from build123d import *

# Parameters (mm, degrees)
F0_R     = 3.96875
F1_DEPTH = 12.7
F4_DEPTH = 12.7
F6_DEPTH = 12.7
F8_DEPTH = 330.2


with BuildPart() as f1:
    # F0 (on Top) → F1 (new body)
    with BuildSketch(Plane.XY):
        Polygon((342.9, 76.2), (-342.9, 76.2), (-377.825, 31.75), (-377.825, -31.75), (-342.9, -76.2), (342.9, -76.2), align=None)
        with Locations((-317.5, -63.5)):
            Circle(F0_R, mode=Mode.SUBTRACT)
        with Locations((-190.5, -63.5)):
            Circle(F0_R, mode=Mode.SUBTRACT)
        with Locations((-63.5, -63.5)):
            Circle(F0_R, mode=Mode.SUBTRACT)
        with Locations((63.5, -63.5)):
            Circle(F0_R, mode=Mode.SUBTRACT)
        with Locations((190.5, -63.5)):
            Circle(F0_R, mode=Mode.SUBTRACT)
        with Locations((317.5, -63.5)):
            Circle(F0_R, mode=Mode.SUBTRACT)
        with Locations((-317.5, 63.5)):
            Circle(F0_R, mode=Mode.SUBTRACT)
        with Locations((-190.5, 63.5)):
            Circle(F0_R, mode=Mode.SUBTRACT)
        with Locations((-63.5, 63.5)):
            Circle(F0_R, mode=Mode.SUBTRACT)
        with Locations((63.5, 63.5)):
            Circle(F0_R, mode=Mode.SUBTRACT)
        with Locations((190.5, 63.5)):
            Circle(F0_R, mode=Mode.SUBTRACT)
        with Locations((317.5, 63.5)):
            Circle(F0_R, mode=Mode.SUBTRACT)
    extrude(amount=F1_DEPTH)

    # F3 (on plane+point) → F4 (join)
    with BuildSketch(Plane.YZ.offset(-342.9)):
        Polygon((76.2, 63.5), (-76.2, 63.5), (-76.2, 12.7), (-31.75, 12.7), (-31.75, 50.8), (31.75, 50.8), (31.75, 12.7), (76.2, 12.7), align=None)
    extrude(amount=F4_DEPTH)

    # F5 (on face) → F6 (join)
    with BuildSketch(Plane.YZ.offset(342.9)):
        Polygon((-76.2, 63.5), (-76.2, 12.7), (-31.75, 12.7), (-31.75, 50.8), (31.75, 50.8), (31.75, 12.7), (76.2, 12.7), (76.2, 63.5), align=None)
    extrude(amount=-F6_DEPTH)

    # F7 (on Right) → F8 (join, symmetric)
    with BuildSketch(Plane.YZ):
        Polygon((69.85, 12.7), (76.2, 12.7), (76.2, 57.15), (71.4375, 57.15), (71.4375, 55.5625), (74.6125, 55.5625), (74.6125, 44.45), (69.85, 44.45), align=None)
        Polygon((-71.4375, 57.15), (-76.2, 57.15), (-76.2, 12.7), (-69.85, 12.7), (-69.85, 44.45), (-74.6125, 44.45), (-74.6125, 55.5625), (-71.4375, 55.5625), align=None)
    extrude(amount=F8_DEPTH, both=True)


solid = f1.part
For this review, take the finished solid that the model builds, in its own axes (mm). A direction names the side the tool comes from. Round coordinates to 2 decimals unless told otherwise and drop trailing zeros. Write each loop counter-clockwise with the first axis right and the second up, starting at its lowest first coordinate (ties: lowest second). Pieces come first, ordered by that corner, then holes. Notation, with made-up numbers: (58, -18.75) - (111, -18.75) arc R10 cw to (111, -9.75) - close; hole circle Ø4 at (-11.75, 58). An arc over 180 degrees is marked (long way). Use a Markdown table: item, result.
Q1. The part is to be moulded in two halves that separate along X. For faces 1 (the flat face through (330.2, -1, 55)), 2 (the flat face through (337, 0, 50.8)), 3 (the flat face through (-360.61, -53.66, 6.26)), say which applies: pulls with the +X half, pulls with the -X half, needs draft (parallel to the pull), parting line crosses it, or undercut.
Derived:
| item | result |
|---|---|
| face 1 | undercut |
| face 2 | needs draft |
| face 3 | pulls with the -X half |
Q2. We need section C-C (x = -261). Give the boundary of the cut face in (y, z), plus the area to 3 significant figures.
Derived:
| item | result |
|---|---|
| outline | (-76.2, 0) - (76.2, 0) - (76.2, 57.15) - (71.44, 57.15) - (71.44, 55.56) - (74.61, 55.56) - (74.61, 44.45) - (69.85, 44.45) - (69.85, 12.7) - (-69.85, 12.7) - (-69.85, 44.45) - (-74.61, 44.45) - (-74.61, 55.56) - (-71.44, 55.56) - (-71.44, 57.15) - (-76.2, 57.15) - close |
| area | 2,390 mm2 |
Q3. Machinability: for faces 4 (the flat face through (5, -69.85, 28)), 5 (the flat face through (-337, 1, 63.5)), 6 (the flat face through (-337, 0, 50.8)), 7 (the flat face through (-342.9, -1, 55)), 8 (the flat face through (5, -74.612, 50)), which of the approach directions +Z, -Z, +X, -X, +Y, -Y give a long, thin tool a straight path to every point of the face, cutting with its end or side? Answer none if there is none.
Derived:
| item | result |
|---|---|
| face 4 | +Z |
| face 5 | +Z, +X, -X, +Y, -Y |
| face 6 | +X, -X |
| face 7 | +Z, -X, +Y, -Y |
| face 8 | none |
Q4. We need section B-B (y = -23). Give the boundary of the cut face in (x, z) (3 decimals).
Derived:
| item | result |
|---|---|
| outline | (-377.825, 0) - (342.9, 0) - (342.9, 12.7) - (-377.825, 12.7) - close; (-342.9, 50.8) - (-330.2, 50.8) - (-330.2, 63.5) - (-342.9, 63.5) - close; (330.2, 50.8) - (342.9, 50.8) - (342.9, 63.5) - (330.2, 63.5) - close |
Q5. We need section A-A (z = 6). State how many separate pieces and enclosed holes the cut face has, plus the area to 3 significant figures.
Derived:
| item | result |
|---|---|
| separate pieces | 1 |
| enclosed holes | 12 |
| area | 108,000 mm2 |
Q6. Wall thickness on line 1 along Y through (x, z) = (-63, 3); line 2 along Y through (x, z) = (304.5, 13); line 3 along Y through (x, z) = (-18.5, 47): over which ranges is each line inside the solid? List them lowest first.
Derived:
| item | result |
|---|---|
| line 1 | y = -76.2 to -67.44, -59.56 to 59.56, 67.44 to 76.2 |
| line 2 | y = -76.2 to -69.85, 69.85 to 76.2 |
| line 3 | y = -76.2 to -74.61, 74.61 to 76.2 |
Q7. Clearance check with flat-ended pins moving along their axes: pin 1 (10.5 mm diameter, centred on x = -190.5, y = 63.5, fed in from +Z); pin 2 (2.5 mm diameter, centred on x = -129, y = 73.5, fed in from +Z). State where each tip first meets the part, or that it passes through.
Derived:
| item | result |
|---|---|
| pin 1 | stops at z = 12.7 |
| pin 2 | stops at z = 57.15 |
